Autodesk Inventor part; units mm, degrees
ref_plane "YZ Plane" through (0, 0, 0) normal (1, 0, 0) x (0, 1, 0)
ref_plane "XZ Plane" through (0, 0, 0) normal (0, 1, 0) x (-1, 0, 0)
ref_plane "XY Plane" through (0, 0, 0) normal (0, 0, 1) x (1, 0, 0)
sketch "Sketch1" plane through (0, 0, 0) normal (0, 1, 0) x (-1, 0, 0)
  line L0 (15, 14.965) -> (-15, 14.965)
  line L1 (-15, 14.965) -> (-15, -14.965)
  line L2 (-15, -14.965) -> (15, -14.965)
  line L3 (15, -14.965) -> (15, 14.965)
  point P0 (0, 0)
  dimension "d0" = 29.93
  dimension "d1" = 30
  dimension "d2" = 15
  dimension "d3" = 14.965
extrude "Plate1" add sketch "Sketch1" along normal blind 1.5
sketch "Sketch2" plane through (-15, 0, -13.465) normal (0, 0, -1) x (-1, 0, 0)
  line L0 (-30, 0) -> (0, 0)
  line L1 (0, 0) -> (0, 43)
  line L2 (0, 43) -> (-30, 43)
  line L3 (-30, 43) -> (-30, 0)
edge flange "Flange1" height 43 angle 90 thickness 1.5 bend radius 0.31 thickness toward (0, 0, -1) relief tear relief width 1.5 relief depth 0.75 corner gap 0.31 corner form 0 edges at (0, 1.5, -14.965) (0, 1.5, 14.965) wall of the first edge with corners at (15, 0, -13.465) (-15, 0, -13.465) (-15, 43, -13.465) (15, 43, -13.465)
bend "Bend1"
corner "Corner1"
sketch "Sketch3" plane through (-15, 43, 14.965) normal (0, 0, 1) x (1, 0, 0)
  line L0 (0, 0) -> (30, 0)
  line L1 (0, -41.19) -> (0, 0)
  circle A0 centre (15, -10) radius 10
  line L2 (0, -18.5) -> (30, -18.5)
  line L3 (30, -18.5) -> (30, -28.5)
  line L4 (30, -28.5) -> (0, -28.5)
  line L5 (0, -28.5) -> (0, -18.5)
  line L6 (30, -18.5) -> (24.0624, -5.7723)
  line L7 (0, -18.5) -> (5.9376, -5.7723)
  line L8 (0, 0) -> (30, 0)
  line L9 (30, 0) -> (30, -25)
  line L10 (30, -25) -> (0, -25)
  line L11 (0, -25) -> (0, 0)
  point P0 (15, -43)
  point P1 (15, 0)
  dimension "d15" = 10
  dimension "d16" = 0
  dimension "d17" = 20
  dimension "d18" = 8.5
  dimension "d19" = 0
  dimension "d20" = 30
  dimension "d21" = 10
  dimension "d22" = 25
extrude "Extrusion1" cut sketch "Sketch3" against normal blind 35 contours L0 A0 L7 L1 | L0 L9 L6 A0
sketch "Sketch4" plane through (15, 1.81, -14.965) normal (0, 0, -1) x (-1, 0, 0)
  arc A0 (24.0624, 35.4177) -> (5.9376, 35.4177) centre (15, 31.19) ccw
  circle A1 centre (15, 31.19) radius 2.6
  circle A2 centre (8, 31.19) radius 1.05
  circle A3 centre (22, 31.19) radius 1.05
  circle A4 centre (15, 38.19) radius 1.05
  circle A5 centre (15, 24.19) radius 1.05
  point P0 (15, -1.81)
  dimension "d25" = 5.2
  dimension "d26" = 0
  dimension "d27" = 7
  dimension "d28" = 2.1
  dimension "d29" = 7
  dimension "d30" = 0
  dimension "d31" = 2.1
  dimension "d32" = 0
  dimension "d33" = 7
  dimension "d34" = 2.1
  dimension "d35" = 7
  dimension "d36" = 0
  dimension "d37" = 2.1
extrude "Extrusion2" cut sketch "Sketch4" against normal blind 1.5
sketch "Sketch5" plane through (-15, 1.81, 14.965) normal (0, 0, 1) x (1, 0, 0)
  arc A0 (24.0624, 35.4177) -> (5.9376, 35.4177) centre (15, 31.19) ccw
  circle A1 centre (15, 31.19) radius 2.5
  point P0 (15, -1.81)
  dimension "d40" = 5
extrude "Extrusion3" cut sketch "Sketch5" against normal blind 1.5
equation "\"d4\" = Thickness"
equation "\"d5\" = BendReliefWidth"
equation "\"d6\" = BendReliefDepth"
equation "\"d7\" = MinimumRemnant"
equation "\"d8\" = TransitionRadius"
equation "\"d11\" = BendRadius"
equation "\"d12\" = CornerReliefSize"
equation "\"d13\" = GapSize"
equation "\"d14\" = JacobiRadiusSize"
equation "\"BendReliefWidth\" = Thickness"
equation "\"BendReliefDepth\" = 0.5 * Thickness"
equation "\"CornerReliefSize\" = 4 * Thickness"
equation "\"MinimumRemnant\" = 2 * Thickness"
equation "\"TransitionRadius\" = BendRadius"
equation "\"JacobiRadiusSize\" = BendRadius"
equation "\"GapSize\" = Thickness"
properties part number "partpart" material "Aluminum 6061-AHC"
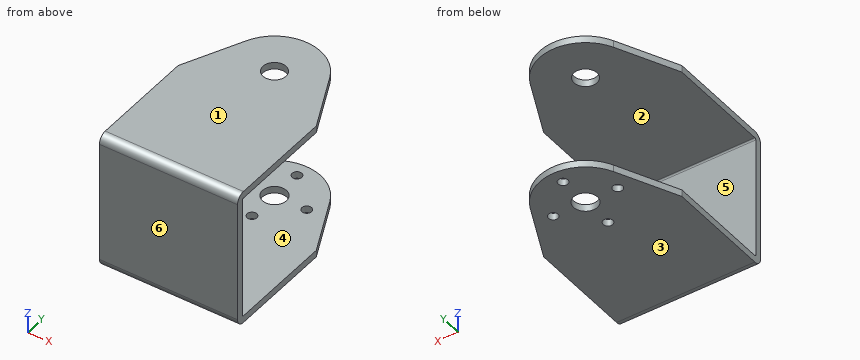
Work out the finished part from the listing and answer in its coordinate system (mm). Face numbers are marked on the shaded views. A direction names the side the tool comes from. Give positions to 0.01 mm unless a question says otherwise; leave off trailing zeros. Loops run counter-clockwise (first coordinate to the right, second up) from the corner with the lowest first, then second, coordinate; pieces in that order, holes last. Notation, with made-up numbers: (60, 9.5) - (69, 9.5) arc R15 cw to (69, 34.5) - close; hole circle Ø8 at (7, 33.5). An arc over 180 degrees is marked (long way). Answer in a Markdown table with one row per item. Add a question column.
Q1. The part is cut by section B-B (y = 18). Determine the outline of the cut face in (x, z) (3 decimals), and give its area (3 significant figures).
Q2. The part is cut by section A-A (x = 0). Determine the outline of the cut face in (y, z) (3 decimals).
Q3. The part is cut by section D-D (y = 26). Determine the outline of the cut face in (x, z) (3 decimals).
Q4. Determine the mould class of the marked faces 1, 2, 3 and 4 for opening direction Z: released by +Z, released by -Z, zero draft, split by the parting line, or undercut.
Q5. A tool of negligible diameter and unlimited length cuts with its end or side. For the marked faces 5 and 6, from which of +Z, -Z, +X, -X, +Y, -Y can it reach the whole face along a straight path? Write none if from no direction.
Q6. Each of these flat-tipped pins is pushed along its axis until it touches: P1, Ø13, axis at x = -4.5, z = 2.5, coming from the +Y side; P2, Ø10, axis at x = -5.5, z = 11.5, coming from the +Y side; P3, Ø1.7, axis at x = 0, y = 26, coming from the -Z side (3 decimals). Where does it stop, or does it pass through?
Q7. The part is cut by section C-C (x = 7). Determine the outline of the cut face in (y, z) (3 decimals).
Q8. Consider line 1 along Z through (x, y) = (-10.5, 33.5) (3 decimals); line 2 along Y through (x, z) = (7, -13.85); line 3 along Y through (x, z) = (7, -14.5). Determine where each line is inside the solid, lowest interval first.
Solution:
| question | item | result |
|---|---|---|
| 1 | outline | (-15, -14.965) - (15, -14.965) - (15, -13.465) - (-15, -13.465) - close; (-15, 13.465) - (15, 13.465) - (15, 14.965) - (-15, 14.965) - close |
| 1 | area | 90.0 mm² |
| 2 | outline | (0, -13.155) arc R1.81 ccw to (1.81, -14.965) - (24.95, -14.965) - (24.95, -13.465) - (1.81, -13.465) arc R0.31 cw to (1.5, -13.155) - (1.5, 13.155) arc R0.31 cw to (1.81, 13.465) - (30.5, 13.465) - (30.5, 14.965) - (1.81, 14.965) arc R1.81 ccw to (0, 13.155) - close; (27.05, -14.965) - (30.4, -14.965) - (30.4, -13.465) - (27.05, -13.465) - close; (35.5, 13.465) - (43, 13.465) - (43, 14.965) - (35.5, 14.965) - close; (35.6, -14.965) - (38.95, -14.965) - (38.95, -13.465) - (35.6, -13.465) - close; (41.05, -14.965) - (43, -14.965) - (43, -13.465) - (41.05, -13.465) - close |
| 3 | outline | (-14.3, -14.965) - (-1.05, -14.965) - (-1.05, -13.465) - (-14.3, -13.465) - close; (-14.3, 13.465) - (14.3, 13.465) - (14.3, 14.965) - (-14.3, 14.965) - close; (1.05, -14.965) - (14.3, -14.965) - (14.3, -13.465) - (1.05, -13.465) - close |
| 4 | face 1 | released by +Z |
| 4 | face 2 | undercut |
| 4 | face 3 | released by -Z |
| 4 | face 4 | undercut |
| 5 | face 5 | +X, -X, +Y |
| 5 | face 6 | +Z, -Z, +X, -X, -Y |
| 6 | P1 | stops at y = 1.5 |
| 6 | P2 | stops at y = 42.96 |
| 6 | P3 | stops at z = 13.465 |
| 7 | outline | (0, -13.155) arc R1.81 ccw to (1.81, -14.965) - (31.95, -14.965) - (31.95, -13.465) - (1.81, -13.465) arc R0.31 cw to (1.5, -13.155) - (1.5, 13.155) arc R0.31 cw to (1.81, 13.465) - (40.141, 13.465) - (40.141, 14.965) - (1.81, 14.965) arc R1.81 ccw to (0, 13.155) - close; (34.05, -14.965) - (40.141, -14.965) - (40.141, -13.465) - (34.05, -13.465) - close |
| 8 | line 1 | z = -14.965 to -13.465, 13.465 to 14.965 |
| 8 | line 2 | y = 0.14 to 31.95, 34.05 to 40.14 |
| 8 | line 3 | y = 0.6 to 31.95, 34.05 to 40.14 |
